```python
from build123d import *

# Parameters (mm, degrees)
SKETCH2_W                = 60
SKETCH2_H                = 60
SKETCH2_W_2              = 48
SKETCH2_H_2              = 48
BOSS_EXTRUDE1_DEPTH      = 35
SKETCH3_R                = 5
CUT_EXTRUDE1_DEPTH       = 76.663729752
CUT_EXTRUDE2_REACH       = 77.664
SKETCH4_R                = 5
BOSS_EXTRUDE2_START      = 2
SKETCH5_R                = 9
SKETCH5_R_2              = 5
BOSS_EXTRUDE2_DEPTH      = 2
BOSS_EXTRUDE3_START      = 2
SKETCH7_R                = 9
SKETCH7_R_2              = 5
BOSS_EXTRUDE3_DEPTH      = 2
BOSS_EXTRUDE4_DEPTH      = 57
BOSS_EXTRUDE4_DEPTH_BACK = 57
SKETCH8_R                = 5
BOSS_EXTRUDE5_DEPTH      = 30
BOSS_EXTRUDE5_DEPTH_BACK = 30
SKETCH9_R                = 5


with BuildPart() as part:
    # Sketch2 → Boss-Extrude1 (new body)
    with BuildSketch(Plane(origin=(0, 0, 0), x_dir=(1, 0, 0), z_dir=(0, 1, 0))):
        Rectangle(SKETCH2_W, SKETCH2_H)
        Rectangle(SKETCH2_W_2, SKETCH2_H_2, mode=Mode.SUBTRACT)
    extrude(amount=BOSS_EXTRUDE1_DEPTH)

    # Sketch3 → Cut-Extrude1 (cut, through all)
    with BuildSketch(Plane(origin=(30, 0, 0), x_dir=(0, 0, -1), z_dir=(1, 0, 0))):
        with Locations((0, 17.5)):
            Circle(SKETCH3_R)
    extrude(amount=-CUT_EXTRUDE1_DEPTH, mode=Mode.SUBTRACT)

    # Sketch4 → Cut-Extrude2 (cut, up to next)
    with BuildSketch(Plane.XY.offset(30), mode=Mode.PRIVATE) as cut_extrude2_sk1:
        with Locations((0, 17.5)):
            Circle(SKETCH4_R)
    cut_extrude2_tool1 = extrude(cut_extrude2_sk1.sketch, amount=-CUT_EXTRUDE2_REACH, mode=Mode.PRIVATE) & part.part
    add(cut_extrude2_tool1.solids().sort_by_distance((0, 17.5, 30))[0], mode=Mode.SUBTRACT)

    # Sketch5 → Boss-Extrude2 (add)
    with BuildSketch(Plane.XY.offset(30).offset(BOSS_EXTRUDE2_START)):
        with Locations(Location((0, 17.5, 0), (0, 0, 180))):
            Circle(SKETCH5_R)
        with Locations((0, 17.5)):
            Circle(SKETCH5_R_2, mode=Mode.SUBTRACT)
    extrude(amount=-BOSS_EXTRUDE2_DEPTH)

    # Sketch7 → Boss-Extrude3 (add)
    with BuildSketch(Plane(origin=(30, 0, 0), x_dir=(0, 0, -1), z_dir=(1, 0, 0)).offset(BOSS_EXTRUDE3_START)):
        with Locations(Location((0, 17.5, 0), (0, 0, 180))):
            Circle(SKETCH7_R)
        with Locations((0, 17.5)):
            Circle(SKETCH7_R_2, mode=Mode.SUBTRACT)
    boss_extrude3 = extrude(amount=-BOSS_EXTRUDE3_DEPTH)

    # Mirror1: Boss-Extrude3 across plane
    add(boss_extrude3.mirror(Plane(origin=(0, 0, 0), x_dir=(0, 0, 1), z_dir=(1, 0, 0))))

    # Sketch8 → Boss-Extrude4 (add, two sides: drawn at the far end of the back side and taken through both)
    with BuildSketch(Plane(origin=(0, 0, 0), x_dir=(0, 0, -1), z_dir=(1, 0, 0)).offset(-BOSS_EXTRUDE4_DEPTH_BACK)):
        with Locations((0, 17.5)):
            Circle(SKETCH8_R)
    extrude(amount=BOSS_EXTRUDE4_DEPTH + BOSS_EXTRUDE4_DEPTH_BACK)

    # Sketch9 → Boss-Extrude5 (add, two sides: drawn at the far end of the back side and taken through both)
    with BuildSketch(Plane.XY.offset(32).offset(-BOSS_EXTRUDE5_DEPTH_BACK)):
        with Locations(Location((0, 17.5, 0), (0, 0, 293.578178478))):
            Circle(SKETCH9_R)
    extrude(amount=BOSS_EXTRUDE5_DEPTH + BOSS_EXTRUDE5_DEPTH_BACK)


solid = part.part
```
Verification items for the finished model (mm, model axes). A direction names the side the tool comes from. Round coordinates to 2 decimals unless told otherwise and drop trailing zeros. Write each loop counter-clockwise with the first axis right and the second up, starting at its lowest first coordinate (ties: lowest second). Pieces come first, ordered by that corner, then holes.
1. Gauge pin test, flat ends, axial feed: P1, Ø1, axis at x = -19, y = 18.5, coming from the +Z side; P2, Ø8, axis at y = 15, z = 49, coming from the +X side; P3, Ø1, axis at y = 31, z = -1, coming from the -X side; P4, Ø6, axis at y = 27, z = 44.5, coming from the +X side. Record the tip position at first contact, or that the pin passes through.
2. Scan lines: L1, parallel to X at y = 13.5, z = 13.5; L2, parallel to Z at x = -4, y = 28. Record each from-to range of solid material in increasing order.
3. Section check C-C on y = 7. Enter the section's corners in (x, z).
4. Section check D-D on x = 21.5. Enter the section's corners in (y, z).
5. Draft check along X on faces 1 (the flat face through (30, 25, 7)), 2 (the flat face through (-30, 25, 7)), 3 (the cylindrical face through (-44.68, 12.62, 1.08)), 4 (the cylindrical face through (-0.336, 15.585, -4.619)). Enter one of: +X half, -X half, draft (parallel to the pull), parting line (faces both ways), or undercut.
6. Section check A-A on z = -19. Enter the section's corners in (x, y).
7. Access from +Z, -Z, +X, -X, +Y, -Y to the whole of each face (thin tool, end or side, straight path). Record for faces 5 (the flat face through (-32, 21, 4)), 6 (the flat face through (-4, 21, 32)), 7 (the cylindrical face through (31.014, 11.417, -6.633)).
8. Section check B-B on x = 0. Enter the section's corners in (y, z), plus the area to 3 significant figures.
Answer:
1. P1: stops at z = 30
1. P2: stops at x = 5
1. P3: stops at x = -30
1. P4: passes through
2. L1: x = -30 to -24, -3 to 3, 24 to 30
2. L2: z = -30 to -24, 24 to 30
3. outline: (-30, -30) - (30, -30) - (30, 30) - (-30, 30) - close; hole (-24, -24) - (24, -24) - (24, 24) - (-24, 24) - close
4. outline: (0, -30) - (35, -30) - (35, -24) - (0, -24) - close; (0, 24) - (35, 24) - (35, 30) - (0, 30) - close; circle Ø10 at (17.5, 0)
5. face 1: +X half
5. face 2: -X half
5. face 3: draft
5. face 4: undercut
6. outline: (-30, 0) - (-24, 0) - (-24, 35) - (-30, 35) - close; (24, 0) - (30, 0) - (30, 35) - (24, 35) - close
7. face 5: -X
7. face 6: +Z
7. face 7: +X
8. outline: (0, -30) - (35, -30) - (35, -24) - (0, -24) - close; (0, 24) - (12.5, 24) - (12.5, 2) - (12.92, 2) arc R5 ccw (long way) to (22.08, 2) - (22.5, 2) - (22.5, 24) - (35, 24) - (35, 30) - (26.5, 30) - (26.5, 32) - (22.5, 32) - (22.5, 62) - (12.5, 62) - (12.5, 32) - (8.5, 32) - (8.5, 30) - (0, 30) - close
8. area: 1,030 mm2
